Here's how the part is built. I have some questions about the finished solid (model axes, mm). Face numbers are marked on the shaded views. A direction names the side the tool comes from. Give positions to 0.01 mm unless a question says otherwise; leave off trailing zeros. Loops run counter-clockwise (first coordinate to the right, second up) from the corner with the lowest first, then second, coordinate; pieces in that order, holes last.
Q1. I need wall thicknesses on probe 1 along Z at (x, y) = (35, 1.75); probe 2 along X at (y, z) = (10.5, 7.25); probe 3 along Z at (x, y) = (12.5, 1.25). Which ranges of each line are inside material? Lowest first, please.
Q2. For the marked faces 1 and 2, which set-ups out of +Z, -Z, +X, -X, +Y, -Y let a thin tool reach every point of the face, with its end or its side?
Q3. Suppose I cut it at C-C (z = 7.75). List the corners of the cut face in (x, y) for me.
Q4. Suppose I cut it at D-D (y = 12.25). List the corners of the cut face in (x, z) for me, and give its area (3 significant figures).
Q5. Suppose I cut it at B-B (y = 22). List the corners of the cut face in (x, z) for me, and give its area (3 significant figures).
Q6. Suppose I cut it at A-A (x = 5). List the corners of the cut face in (y, z) for me.
Q7. I'm going to push flat-ended pins straight in: P1, Ø1, axis at x = 4.5, y = 22, coming from the +Z side; P2, Ø9.5, axis at y = 11.5, z = 15, coming from the +X side; P3, Ø1.5, axis at x = 5.5, z = 22.5, coming from the +Y side. Where does each tip first touch, or does it pass through?
```python
from build123d import *

# Parameters (mm, degrees)
F0_W     = 38.1
F0_H     = 25.4
F1_DEPTH = 25.4
F3_DEPTH = 38.101
F4_DEPTH = 38.101
F5_DEPTH = 25.4


with BuildPart() as f1:
    # F0 (on Top) → F1 (new body)
    with BuildSketch(Plane.XY):
        with Locations((19.05, 12.7)):
            Rectangle(F0_W, F0_H)
    extrude(amount=F1_DEPTH)

    # F2 (on face) → F3 (cut, through all)
    with BuildSketch(Plane.YZ.offset(38.1)):
        with BuildLine():
            ThreePointArc((12.7, 25.4), (21.6802561211, 21.6802561211), (25.4, 12.7))
            Line((25.4, 12.7), (25.4, 25.4))
            Line((25.4, 25.4), (12.7, 25.4))
        make_face()
        with BuildLine():
            ThreePointArc((0, 12.7), (3.7197438789, 21.6802561211), (12.7, 25.4))
            Line((12.7, 25.4), (0, 25.4))
            Line((0, 25.4), (0, 12.7))
        make_face()
    extrude(amount=-F3_DEPTH, mode=Mode.SUBTRACT)

    # F2 (on face) → F4 (cut, through all)
    with BuildSketch(Plane.YZ.offset(38.1)):
        with BuildLine():
            ThreePointArc((12.7, 25.4), (21.6802561211, 21.6802561211), (25.4, 12.7))
            Line((25.4, 12.7), (25.4, 25.4))
            Line((25.4, 25.4), (12.7, 25.4))
        make_face()
    extrude(amount=-F4_DEPTH, mode=Mode.SUBTRACT)

    # F2 (on face) → F5 (cut)
    with BuildSketch(Plane.YZ.offset(38.1)):
        with BuildLine():
            Line((25.4, 6.35), (25.4, 12.7))
            ThreePointArc((25.4, 12.7), (21.6802561211, 21.6802561211), (12.7, 25.4))
            ThreePointArc((12.7, 25.4), (3.7197438789, 21.6802561211), (0, 12.7))
            Line((0, 12.7), (0, 6.35))
            Line((0, 6.35), (25.4, 6.35))
        make_face()
    extrude(amount=-F5_DEPTH, mode=Mode.SUBTRACT)


solid = f1.part
```
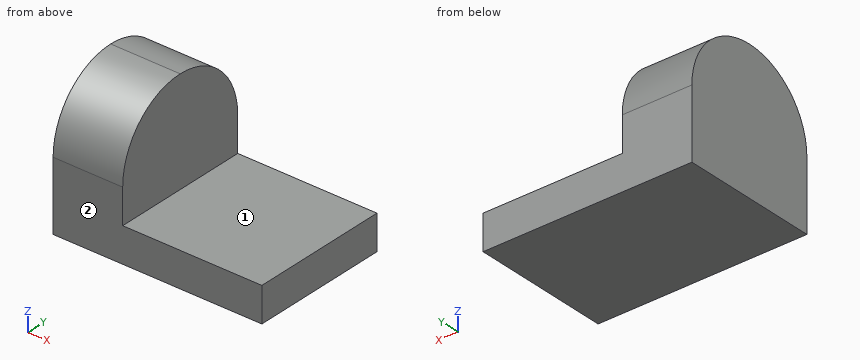
Solutions:
1. probe 1: z = 0 to 6.35
1. probe 2: x = 0 to 12.7
1. probe 3: z = 0 to 18.19
2. face 1: +Z, +X, +Y, -Y
2. face 2: +Z, -Z, +X, -X, -Y
3. outline: (0, 0) - (12.7, 0) - (12.7, 25.4) - (0, 25.4) - close
4. outline: (0, 0) - (38.1, 0) - (38.1, 6.35) - (12.7, 6.35) - (12.7, 25.39) - (0, 25.39) - close
4. area: 484 mm2
5. outline: (0, 0) - (38.1, 0) - (38.1, 6.35) - (12.7, 6.35) - (12.7, 21.35) - (0, 21.35) - close
5. area: 432 mm2
6. outline: (0, 0) - (25.4, 0) - (25.4, 12.7) arc R12.7 ccw to (0, 12.7) - close
7. P1: stops at z = 21.86
7. P2: stops at x = 12.7
7. P3: stops at y = 21.61
